The listing builds one solid part. Answer for the finished solid, in the listing's coordinates (mm). Face numbers are marked on the shaded views. A direction names the side the tool comes from. Coordinates: 2 decimals unless noted, no trailing zeros. Order: outer loops, then holes, each group sorted by start corner. A loop starts at its lowest first (then second) coordinate and runs counter-clockwise, first axis right, second up. Notation, with made-up numbers: M 57,11.25 L 99,11.25 A17 ccw 99,15.25 Z; hole C 4,52 d3. An arc over 180 degrees is marked long. One line per item, written item: value. Start each with the question number.
Q1. The part is cut by section A-A on z = 21. Give the vertices of the cut face in (x, y).
Q2. Determine the mould class of the marked faces 1, 2, 3 and 4 for opening direction X: pulls with the +X half, pulls with the -X half, needs draft (parallel to the pull), parting line crosses it, or undercut.
Q3. For the marked faces 5 and 6, determine the directions among +Z, -Z, +X, -X, +Y, -Y from which every point of the face is accessible in a straight line to the end or side of a thin tool.
Q4. Straight lines are drawn through the part: line 1 along Z through (x, y) = (-27.5, 16.5); line 2 along X through (y, z) = (11.25, 7); line 3 along Z through (x, y) = (-30, 16.5). For each, find the intervals that lie inside material, in ascending order. Write a range as [from, to].
Q5. This flat-tipped pin is pushed along its axis until it touches: pin 1 Ø3.5 at (x, y) = (-20.62, 13.06) entering from -Z. Where does it stop, or does it pass through?
Q6. The part is cut by section B-B on y = 9.25. Give the vertices of the cut face in (x, z).
Q7. The part is cut by section C-C on z = 8. Give the vertices of the cut face in (x, y), then the cut area to 3 significant figures.
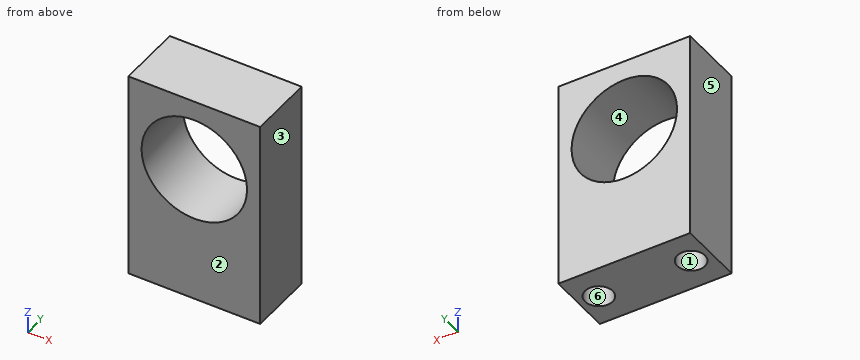
```python
from build123d import *

# Parameters (mm, degrees)
F0_W     = 20
F0_H     = 10
F1_DEPTH = 32
F2_R     = 8
F3_DEPTH = 25
F5_D     = 4.2
F5_DEPTH = 10.4
F5_TIP   = 1.2618073


with BuildPart() as f1:
    # F0 (on Top) → F1 (new body)
    with BuildSketch(Plane.XY):
        with Locations((-27.6177362539, 13.0586402248)):
            Rectangle(F0_W, F0_H)
    extrude(amount=F1_DEPTH)

    # F2 (on face) → F3 (cut)
    with BuildSketch(Plane.XZ.offset(-8.0586402248)):
        with Locations((-27.6177362539, 21)):
            Circle(F2_R)
    extrude(amount=-F3_DEPTH, mode=Mode.SUBTRACT)

    # F5
    with Locations(Plane(origin=(0, 0, 0), x_dir=(1, 0, 0), z_dir=(0, 0, -1))):
        with Locations((-34.6177362539, -13.0586402248), (-20.6177362539, -13.0586402248)):
            Hole(F5_D / 2, depth=F5_DEPTH)
            with Locations((0, 0, -(F5_DEPTH + F5_TIP / 2))):  # 118° drill point
                Cone(0, F5_D / 2, F5_TIP, mode=Mode.SUBTRACT)


solid = f1.part
```
Output:
1. outline: M -37.62,8.06 L -35.62,8.06 L -35.62,18.06 L -37.62,18.06 Z; M -19.62,8.06 L -17.62,8.06 L -17.62,18.06 L -19.62,18.06 Z
2. face 1: undercut
2. face 2: needs draft
2. face 3: pulls with the +X half
2. face 4: undercut
3. face 5: +Z, -Z, -X, +Y, -Y
3. face 6: -Z
4. line 1: z = [0, 13], [29, 32]
4. line 2: x = [-37.62, -35.68], [-33.55, -21.68], [-19.55, -17.62]
4. line 3: z = [0, 13.36], [28.64, 32]
5. pin 1: stops at z = 10.61
6. outline: M -37.62,0 L -17.62,0 L -17.62,32 L -37.62,32 Z; hole C -27.62,21 d16
7. outline: M -37.62,8.06 L -17.62,8.06 L -17.62,18.06 L -37.62,18.06 Z; hole C -34.62,13.06 d4.2; hole C -20.62,13.06 d4.2
7. area: 172 mm^2
